The drawing under review shows one solid part. Ordinate dimensions are in mm from its lowest x, y, z. A direction names the side the tool comes from. Give positions to 0.01 mm unless a question says otherwise; leave off trailing zeros. Loops run counter-clockwise (first coordinate to the right, second up) from the corner with the lowest first, then second, coordinate; pieces in that order, holes last. Notation, with made-up numbers: (28.5, -13) - (63.5, -13) arc R32 ccw to (63.5, 19) - close; hole circle Ø10 at (28, 60). An arc over 180 degrees is marked (long way). Write each question's results on one line, items separated by ' | '.
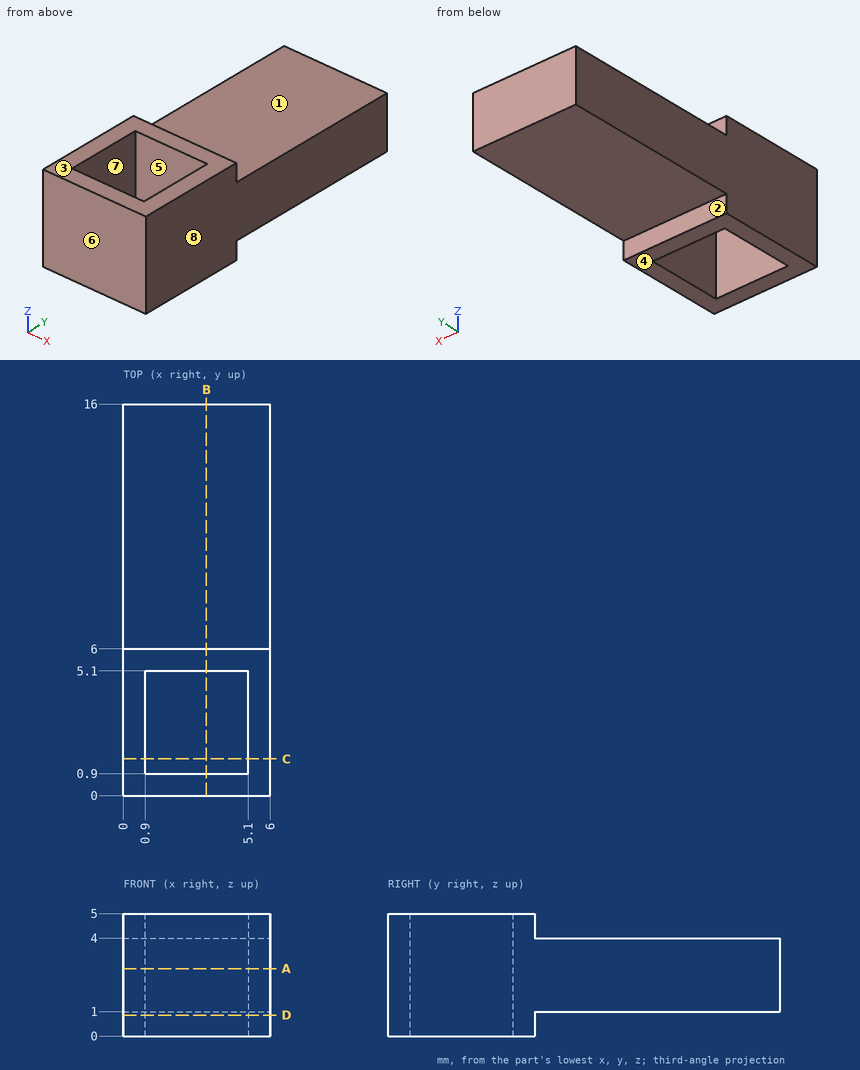
(1) Take a section at B-B on x = 3.4. Give the boundary of the cut face in (y, z), plus the area to 3 significant figures.
Answers below:
outline: (0, 0) - (0.9, 0) - (0.9, 5) - (0, 5) - close; (5.1, 0) - (6, 0) - (6, 1) - (16, 1) - (16, 4) - (6, 4) - (6, 5) - (5.1, 5) - close | area: 39.0 mm2
(2) Take a section at C-C on y = 1.5. Give the boundary of the cut face in (x, z), plus the area to 3 significant figures.
Answers below:
outline: (0, 0) - (0.9, 0) - (0.9, 5) - (0, 5) - close; (5.1, 0) - (6, 0) - (6, 5) - (5.1, 5) - close | area: 9.00 mm2
(3) Tool access review of the marked faces 1, 2, 3, 4 and 5: name each direction out of +Z, -Z, +X, -X, +Y, -Y from which nothing blocks a thin tool from reaching the whole face with its end or side.
Answers below:
face 1: +Z, +X, -X, +Y | face 2: -Z, +X, -X, +Y | face 3: +Z, +X, -X, +Y, -Y | face 4: -Z, +X, -X, +Y, -Y | face 5: +Z, -Z
(4) Wall thickness on line 1 along Y through (x, z) = (4.15, 2.35); line 2 along Y through (x, z) = (2.75, 4.5): over which ranges is each line inside the solid? List them lowest first. Write a range as from..to.
Answers below:
line 1: 0..0.9, 5.1..16 | line 2: 0..0.9, 5.1..6
(5) Draft analysis for pull direction X (two halves, no side actions). For the marked faces 6, 7 and 8, state which applies: pulls with the +X half, pulls with the -X half, needs draft (parallel to the pull), parting line crosses it, or undercut.
Answers below:
face 6: needs draft | face 7: undercut | face 8: pulls with the +X half
(6) Take a section at A-A on z = 2.75. Give the boundary of the cut face in (x, y), plus the area to 3 significant figures.
Answers below:
outline: (0, 0) - (6, 0) - (6, 16) - (0, 16) - close; hole (0.9, 0.9) - (5.1, 0.9) - (5.1, 5.1) - (0.9, 5.1) - close | area: 78.4 mm2
(7) Insertion check: P1, Ø1.8, axis at x = 3, y = 11, coming from the -Z side; P2, Ø0.8, axis at x = 4.5, z = 0.5, coming from the +Y side. Each pin has a flat end and moves straight along its axis. Give the tip position at first contact, or say it passes through.
Answers below:
P1: z = 1 | P2: y = 6
(8) Take a section at D-D on z = 0.85. Give the boundary of the cut face in (x, y).
Answers below:
outline: (0, 0) - (6, 0) - (6, 6) - (0, 6) - close; hole (0.9, 0.9) - (5.1, 0.9) - (5.1, 5.1) - (0.9, 5.1) - close
